CAD build for the part. Positions are in the model's coordinates, mm. A direction names the side the tool comes from. Round coordinates to 2 decimals unless told otherwise and drop trailing zeros. Write each loop counter-clockwise with the first axis right and the second up, starting at its lowest first coordinate (ties: lowest second). Pieces come first, ordered by that corner, then holes. Notation, with made-up numbers: (6, 4.5) - (63, 4.5) arc R21 ccw to (63, 42.5) - close; hole circle Ø4 at (11, 87.25). An arc over 180 degrees is marked (long way). Answer in a Markdown table with one row per item.
```python
from build123d import *

# Parameters (mm, degrees)
F3_D           = 2.7
F3_CBORE_D     = 4.5
F3_CBORE_DEPTH = 3
F5_D           = 2.7
F5_DEPTH       = 3
F5_TIP         = 0.8111618357
F7_W           = 12.7133149276
F7_H           = 0.9999985352


# Not quite as in the source:
# - a pattern or mirror of a feature is missing from the dataset's text; its kind, count and spacing are read off the source's solid


with BuildPart() as f1:
    # F0 (on Front) → F1 (revolve)
    with BuildSketch(Plane.XZ):
        with BuildLine():
            Line((9.5, 22), (9, 22))
            Line((9, 22), (9, 12))
            Line((9, 12), (9.5, 11.5))
            Line((9.5, 11.5), (9.5, 10.5))
            Line((9.5, 10.5), (9, 10))
            Line((9, 10), (2, 10))
            Line((2, 10), (2, 6))
            Line((2, 6), (2.5, 6))
            Line((2.5, 6), (2.5, 0))
            Line((2.5, 0), (3.5, 0))
            Line((3.5, 0), (3.5, 3))
            Line((3.5, 3), (3.15, 3))
            Line((3.15, 3), (3.15, 4))
            Line((3.15, 4), (11, 4))
            Line((11, 4), (11, 5.5))
            Line((11, 5.5), (10.5, 5.5))
            Line((10.5, 5.5), (10.5, 12.5))
            Line((10.5, 12.5), (11.35, 12.5))
            Line((11.35, 12.5), (11.35, 14.5))
            Line((11.35, 14.5), (10, 14.5))
            Line((10, 14.5), (10, 15.5))
            Line((10, 15.5), (10.5, 15.5))
            Line((10.5, 15.5), (10.5, 18))
            Line((10.5, 18), (10, 18))
            Line((10, 18), (10, 21.5))
            ThreePointArc((10, 21.5), (9.8535533906, 21.8535533906), (9.5, 22))
        make_face()
    revolve(axis=Axis((0, 0, 11), (0, 0, 1)))

    # F3 (through all)
    with Locations(Plane(origin=(0, 0, 4), x_dir=(1, 0, 0), z_dir=(0, 0, -1))):
        with Locations((0, -5.75), (0, 5.75)):
            CounterBoreHole(F3_D / 2, F3_CBORE_D / 2, F3_CBORE_DEPTH)

    # F5
    with Locations(Plane.XY.offset(10)):
        with Locations((3, -3), (3, 3)):
            Hole(F5_D / 2, depth=F5_DEPTH)
            with Locations((0, 0, -(F5_DEPTH + F5_TIP / 2))):  # 118° drill point
                Cone(0, F5_D / 2, F5_TIP, mode=Mode.SUBTRACT)

    # F7 (on face) → F8 (revolve, cut)
    with BuildSketch(Plane(origin=(0, 0, 0), x_dir=(-0.7071067812, -0.7071067812, 0), z_dir=(-0.7071067812, 0.7071067812, 0))):
        with Locations((-10.5992981509, 8.4999992676)):
            Rectangle(F7_W, F7_H)
    f8 = revolve(axis=Axis((7.4948355983, 7.4948355983, 8), (0.7071067812, 0.7071067812, 0)), mode=Mode.SUBTRACT)

    # F8_copies: F8 across plane
    add(f8.mirror(Plane(origin=(0, -1.1e-05, 0), x_dir=(-1, -1e-06, 0), z_dir=(1e-06, -1, 0))), mode=Mode.SUBTRACT)


solid = f1.part
```
Q1. Pull direction Y, two halves, no side cores. Call faces 5 (the cylindrical face through (-2.5, -1.917, 3.507)), 6 (the flat face through (3, -2, 4)), 7 (the cylindrical face through (-0.29, 3.52, 5.48)): released by +Y, released by -Y, zero draft, split by the parting line, or undercut.
Computed:
| item | result |
|---|---|
| face 5 | split by the parting line |
| face 6 | zero draft |
| face 7 | undercut |
Q2. Saw through at D-D on z = 8.25. List the corners of the cut face in (x, y), then the cut area to 3 significant figures.
Computed:
| item | result |
|---|---|
| outline | (2.98, -4.35) arc R1.35 cw (long way) to (4.35, -2.98) - (8.08, -6.71) arc R10.5 ccw to (8.08, 6.71) - (4.35, 2.98) arc R1.35 cw (long way) to (2.98, 4.35) - (6.71, 8.08) arc R10.5 ccw (long way) to (6.71, -8.08) - close; hole circle Ø4 at (0, 0); hole circle Ø2.7 at (0, -5.75); hole circle Ø2.7 at (0, 5.75) |
| area | 291 mm2 |
Q3. Saw through at A-A on z = 4.5. List the corners of the cut face in (x, y).
Computed:
| item | result |
|---|---|
| outline | circle Ø22 at (0, 0); hole circle Ø5 at (0, 0); hole circle Ø4.5 at (0, -5.75); hole circle Ø4.5 at (0, 5.75) |
Q4. 3-axis set-ups, long thin cutter, end or side, ignore diameter. For faces 1 (the cylindrical face through (4.38, -8.43, 10.99)), 2 (the cylindrical face through (0.176, -7.089, 8.521)), 3 (the flat face through (1, 2, 6)), 4 (the cylindrical face through (2.274, -1.862, 8.479)): which of +Z, -Z, +X, -X, +Y, -Y reach the whole face in a straight line?
Computed:
| item | result |
|---|---|
| face 1 | none |
| face 2 | +Z, -Z |
| face 3 | -Z |
| face 4 | +Z |
Q5. Flat gauge pins, fed straight in: pin 1 (6 mm diameter, centred on x = 0, y = 0, fed in from -Z); pin 2 (5 mm diameter, centred on x = 5.5, z = 11, fed in from +Y); pin 3 (5 mm diameter, centred on x = 0, y = -5.75, fed in from +Z); pin 4 (3 mm diameter, centred on x = -8, z = 3.5, fed in from -Y). Where does each tip first touch, or does it go through?
Computed:
| item | result |
|---|---|
| pin 1 | stops at z = 0 |
| pin 2 | stops at y = 10.8 |
| pin 3 | stops at z = 10 |
| pin 4 | stops at y = -8.81 |
Q6. Drill centre lines: line 1 (Y direction, x = 0, z = 9.2); line 2 (Y direction, x = 0, z = 5); line 3 (Z direction, x = -6, y = 8.5). Where is each one in solid material? Low to high.
Computed:
| item | result |
|---|---|
| line 1 | y = -10.5 to -7.1, -4.4 to -2, 2 to 4.4, 7.1 to 10.5 |
| line 2 | y = -11 to -8, -3.5 to -2.5, 2.5 to 3.5, 8 to 11 |
| line 3 | z = 4 to 14.5, 15.5 to 18 |
Q7. Saw through at B-B on x = 0. Count the separate pieces of the cut face and the enclosed holes in it, then the cut area to 3 significant figures.
Computed:
| item | result |
|---|---|
| separate pieces | 4 |
| enclosed holes | 0 |
| area | 98.4 mm2 |
